Can you work these out from the drawing? Everything is in mm from the part's minimum corner. A direction names the side the tool comes from. Round coordinates to 2 decimals unless told otherwise and drop trailing zeros. Loops run counter-clockwise (first coordinate to the right, second up) from the corner with the lowest first, then second, coordinate; pieces in that order, holes last. Notation, with made-up numbers: (51, -22.75) -> (70, -22.75) arc R29 ccw to (70, 3.25) -> close; hole circle Ø2 at (-39, 27). An arc over 180 degrees is marked (long way). Answer as a JSON object with one key per item and string values.
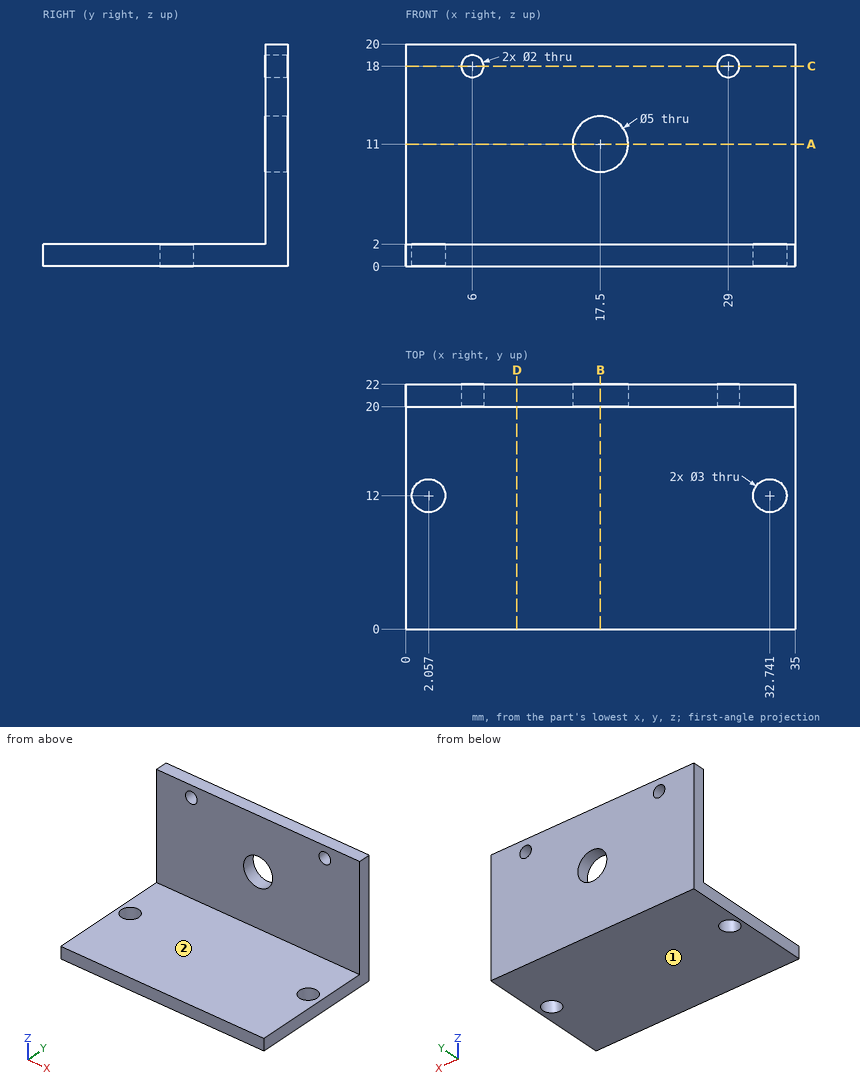
Q1. I'm going to push flat-ended pins straight in: pin 1 (10 mm diameter, centred on x = 24.5, y = 8, fed in from +Z); pin 2 (9 mm diameter, centred on x = 26, z = 10, fed in from -Y). Where does each tip first touch, or does it pass through?
Determined:
{"pin 1": "z = 2", "pin 2": "y = 20"}
Q2. I want a section at A-A, the plane z = 11. Write out the boundary of the cut face in (x, y).
Determined:
{"outline": "(0, 20) -> (15, 20) -> (15, 22) -> (0, 22) -> close; (20, 20) -> (35, 20) -> (35, 22) -> (20, 22) -> close"}
Q3. If I drill on L1, parallel to X at y = 20.7, z = 18; L2, parallel to X at y = 21.4, z = 11; L3, parallel to Z at x = 17, y = 19.25, over which ranges is the centre line in solid material (lowest first)? Write a range as [from, to].
Determined:
{"L1": "[0, 5], [7, 28], [30, 35]", "L2": "[0, 15], [20, 35]", "L3": "[0, 2]"}
Q4. I want a section at B-B, the plane x = 17.5. Write out the boundary of the cut face in (y, z).
Determined:
{"outline": "(0, 0) -> (22, 0) -> (22, 8.5) -> (20, 8.5) -> (20, 2) -> (0, 2) -> close; (20, 13.5) -> (22, 13.5) -> (22, 20) -> (20, 20) -> close"}
Q5. On a 3-axis mill with a long thin cutter (end or side, diameter ignored), from which of +Z, -Z, +X, -X, +Y, -Y can I reach the whole of each face in a straight line? I mean the marked faces 1 and 2. Say none if no direction works.
Determined:
{"face 1": "-Z, +X, -X, +Y, -Y", "face 2": "+Z, +X, -X, -Y"}
Q6. I want a section at C-C, the plane z = 18. Write out the boundary of the cut face in (x, y).
Determined:
{"outline": "(0, 20) -> (5, 20) -> (5, 22) -> (0, 22) -> close; (7, 20) -> (28, 20) -> (28, 22) -> (7, 22) -> close; (30, 20) -> (35, 20) -> (35, 22) -> (30, 22) -> close"}
Q7. I want a section at D-D, the plane x = 10. Write out the boundary of the cut face in (y, z).
Determined:
{"outline": "(0, 0) -> (22, 0) -> (22, 20) -> (20, 20) -> (20, 2) -> (0, 2) -> close"}
